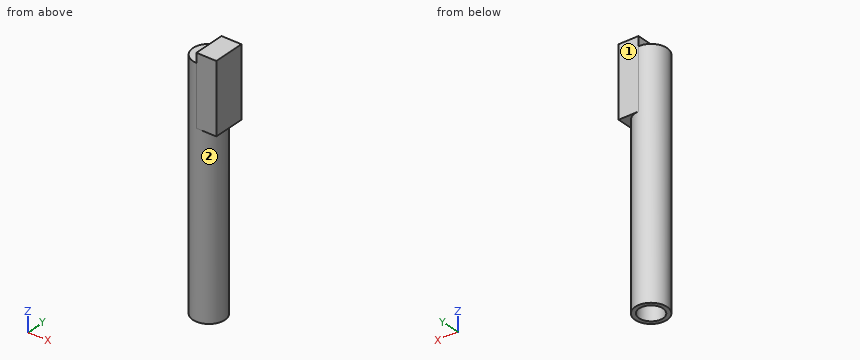
```python
from build123d import *

# Parameters (mm, degrees)
F0_R     = 40
F1_DEPTH = 600
F2_W     = 50
F2_H     = 175
F3_DEPTH = 40
F4_R     = 30
F5_DEPTH = 500


with BuildPart() as f1:
    # F0 (on Top) → F1 (new body)
    with BuildSketch(Plane.XY):
        Circle(F0_R)
    extrude(amount=F1_DEPTH)

    # F2 (on Front) → F3 (join, symmetric)
    with BuildSketch(Plane.XZ):
        with Locations((25, 536.151046)):
            Rectangle(F2_W, F2_H)
    extrude(amount=F3_DEPTH, both=True)

    # F4 (on face) → F5 (cut)
    with BuildSketch(Plane(origin=(0, 0, 0), x_dir=(1, 0, 0), z_dir=(0, 0, -1))):
        Circle(F4_R)
    extrude(amount=-F5_DEPTH, mode=Mode.SUBTRACT)


solid = f1.part
```
Source: CAD feature listing. Evaluate the final solid. Frame: model axes, mm. Face numbers are marked on the shaded views. A direction names the side the tool comes from. Coordinates: 2 decimals unless noted, no trailing zeros. Loops run counter-clockwise (first coordinate to the right, second up) from the corner with the lowest first, then second, coordinate; pieces in that order, holes last. Notation, with made-up numbers: M -27.75,71 L -1.75,71 A9 cw -1.75,83 Z; hole C 53.25,58.5 d9. An arc over 180 degrees is marked long. Put each result on its own line as item: value. Start each with the question number.
1) Ray query, L1, parallel to Y at x = 0, z = 189; L2, parallel to Z at x = 3, y = 4. Return the intervals inside material, ascending. Write a range as from..to.
2) Reachability of the marked faces 1 and 2 from +Z, -Z, +X, -X, +Y, -Y: full face, straight path, thin tool, end or side. Return the list, or none.
3) Contact query for flat-ended pins moving along their axis: pin 1 Ø2 at (x, z) = (21, 217) entering from +Y; pin 2 Ø1.5 at (y, z) = (-17, 327) entering from +X; pin 3 Ø2 at (y, z) = (3.5, 430) entering from +X. Output: stop coordinate, or through.
4) Cut plane C-C on x = 6.5. Return the cut outline in (y, z).
5) Cut plane A-A on z = 465. Return the cut outline in (x, y), then the cut area to 3 significant figures.
6) Cut plane B-B on y = 0. Return the cut outline in (x, z), then the cut area to 3 significant figures.
The answers:
1. L1: y = -40..-30, 30..40
1. L2: z = 500..623.65
2. face 1: +Z, -Z, +X, -X, +Y
2. face 2: -Z
3. pin 1: stops at y = 34.64
3. pin 2: stops at x = 36.55
3. pin 3: stops at x = 39.92
4. outline: M -40,448.65 L -39.47,448.65 L -39.47,0 L -29.29,0 L -29.29,500 L 29.29,500 L 29.29,0 L 39.47,0 L 39.47,448.65 L 40,448.65 L 40,623.65 L -40,623.65 Z
5. outline: M 0,-40 L 50,-40 L 50,40 L 0,40 A40 ccw Z; hole C 0,0 d60
5. area: 3,690 mm²
6. outline: M -40,0 L -30,0 L -30,500 L 30,500 L 30,0 L 40,0 L 40,448.65 L 50,448.65 L 50,623.65 L 0,623.65 L 0,600 L -40,600 Z
6. area: 20,700 mm²
